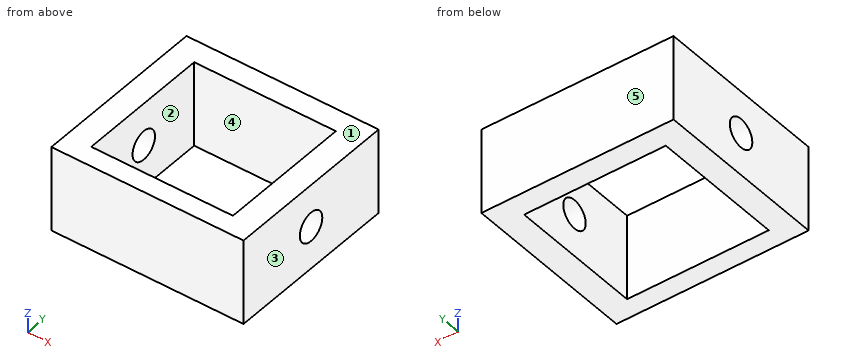
```python
from build123d import *

# Parameters (mm, degrees)
F0_W     = 131.444588
F0_H     = 120.110088
F1_DEPTH = 58.42
F2_R     = 9.981672
F4_DEPTH = 157.226
F5_W     = 96.937245
F5_H     = 91.505859
F6_DEPTH = 129.032


with BuildPart() as f1:
    # F0 (on Top) → F1 (new body)
    with BuildSketch(Plane.XY):
        Rectangle(F0_W, F0_H)
    extrude(amount=F1_DEPTH)

    # F2 (on face) → F4 (cut, symmetric)
    with BuildSketch(Plane.YZ.offset(65.722294)):
        with Locations((0, 29.21)):
            Circle(F2_R)
    extrude(amount=F4_DEPTH, both=True, mode=Mode.SUBTRACT)

    # F5 (on Top) → F6 (cut, symmetric)
    with BuildSketch(Plane.XY):
        with Locations((-0.250232, -0.960483)):
            Rectangle(F5_W, F5_H)
    extrude(amount=F6_DEPTH, both=True, mode=Mode.SUBTRACT)


solid = f1.part
```
Verification items for the finished model (mm, model axes). Face numbers are marked on the shaded views. A direction names the side the tool comes from. Coordinates: 2 decimals unless noted, no trailing zeros. Write each loop counter-clockwise with the first axis right and the second up, starting at its lowest first coordinate (ties: lowest second). Pieces come first, ordered by that corner, then holes. Notation, with made-up numbers: (2, 53) - (22, 53) arc R26 ccw to (22, 67) - close; hole circle Ø10 at (62, 69.5). An arc over 180 degrees is marked (long way). One line per question, with ' | ' between items. Start each with the question number.
1. Section check A-A (y = 42). Enter the section's corners in (x, z).
2. Section check C-C (x = 34). Enter the section's corners in (y, z), plus the area to 3 significant figures.
3. Access from +Z, -Z, +X, -X, +Y, -Y to the whole of each face (thin tool, end or side, straight path). Record for the marked faces 1 and 2.
4. Section check D-D (y = 0). Enter the section's corners in (x, z).
5. Draft check along X on the marked faces 3, 4 and 5. Enter one of: released by +X, released by -X, zero draft, split by the parting line, or undercut.
6. Section check B-B (z = 29.21). Enter the section's corners in (x, y), plus the area to 3 significant figures.
7. Material ranges on line 1 along X through (y, z) = (11.5, 13.5); line 2 along Y through (x, z) = (-55, 29); line 3 along Y through (x, z) = (-29, 47), recorded low to high.
Computed values:
1) outline: (-65.72, 0) - (-48.72, 0) - (-48.72, 58.42) - (-65.72, 58.42) - close; (48.22, 0) - (65.72, 0) - (65.72, 58.42) - (48.22, 58.42) - close
2) outline: (-60.06, 0) - (-46.71, 0) - (-46.71, 58.42) - (-60.06, 58.42) - close; (44.79, 0) - (60.06, 0) - (60.06, 58.42) - (44.79, 58.42) - close | area: 1,670 mm²
3) face 1: +Z, +X, -X, +Y, -Y | face 2: +Z, -Z
4) outline: (-65.72, 0) - (-48.72, 0) - (-48.72, 19.23) - (-65.72, 19.23) - close; (-65.72, 39.19) - (-48.72, 39.19) - (-48.72, 58.42) - (-65.72, 58.42) - close; (48.22, 0) - (65.72, 0) - (65.72, 19.23) - (48.22, 19.23) - close; (48.22, 39.19) - (65.72, 39.19) - (65.72, 58.42) - (48.22, 58.42) - close
5) face 3: released by +X | face 4: undercut | face 5: zero draft
6) outline: (-65.72, -60.06) - (65.72, -60.06) - (65.72, -9.98) - (48.22, -9.98) - (48.22, -46.71) - (-48.72, -46.71) - (-48.72, -9.98) - (-65.72, -9.98) - close; (-65.72, 9.98) - (-48.72, 9.98) - (-48.72, 44.79) - (48.22, 44.79) - (48.22, 9.98) - (65.72, 9.98) - (65.72, 60.06) - (-65.72, 60.06) - close | area: 6,230 mm²
7) line 1: -65.72 to -48.72, 48.22 to 65.72 | line 2: -60.06 to -9.98, 9.98 to 60.06 | line 3: -60.06 to -46.71, 44.79 to 60.06
